Part model, mm, in its own coordinate system. A direction names the side the tool comes from. Coordinates: 2 decimals unless noted, no trailing zeros. Write each loop counter-clockwise with the first axis right and the second up, starting at its lowest first coordinate (ties: lowest second). Pieces come first, ordered by that corner, then holes. Notation, with made-up numbers: (-37.5, -9) -> (8.5, -9) arc R22 cw to (8.5, 12) -> close; hole circle Ø9 at (33, 4). An arc over 180 degrees is marked (long way). One line per question, with ' | ' between items. Start each with the question number.
Item 1: 3-axis set-ups, long thin cutter, end or side, ignore diameter. For faces 1 (the flat face through (77.042, 24.437, 135.393)), 2 (the flat face through (68, 11, 91)): which of +Z, -Z, +X, -X, +Y, -Y reach the whole face in a straight line?
Item 2: Two-plate mould, pull along Y, no slides. Class faces 3 (the cylindrical face through (77.04, 18.35, 147.49)), 4 (the cylindrical face through (77.042, 22.789, 154.427)), 5 (the flat face through (80, 16, 103)): pulls with the +Y half, pulls with the -Y half, needs draft (parallel to the pull), parting line crosses it, or undercut.
Item 3: Saw through at A-A (y = 19.25). List the corners of the cut face in (x, z).
Item 4: Saw through at C-C (y = 25.25). List the corners of the cut face in (x, z), and give its area (3 significant figures).
Item 5: Pin check, flat tips, straight feed: pin 1 (8 mm diameter, centred on x = 63, z = 135.5, fed in from -Y); pin 2 (4 mm diameter, centred on x = 68, z = 115.5, fed in from +Y); pin 3 (12 mm diameter, centred on x = 65, z = 70.5, fed in from -Y); pin 4 (9.5 mm diameter, centred on y = 19.96, z = 144.96, fed in from -X). Stop position of each tip, or through.
Item 6: Probe probe 1 along X at (y, z) = (13, 149); probe 2 along Z at (x, y) = (58.75, 19.75); probe 3 along Y at (x, z) = (64, 130). List the from-to ranges inside material, lowest first. Write a range as [from, to].
Item 7: Saw through at B-B (z = 135.5). List the corners of the cut face in (x, y).
from build123d import *

# Parameters (mm, degrees)
SKETCH014_R      = 3
EXTRUDE013_DEPTH = 6
BOX025_W         = 23
BOX025_H         = 10
BOX025_DEPTH     = 80


with BuildPart() as union_brazo_central:
    # Sketch014 → Extrude013 (new body)
    with BuildSketch(Plane(origin=(0, 0, 0), x_dir=(0, -1, 0), z_dir=(-1, 0, 0))):
        with BuildLine():
            ThreePointArc((-10.900695, 145.407872), (-23.024313, 154.355924), (-27.779278, 140.057671))
            Line((-27.779278, 140.057671), (-20.026942, 129.238365))
            Line((-20.026942, 129.238365), (-11.026942, 129.238365))
            Line((-10.900695, 145.407872), (-11.026942, 129.238365))
        make_face()
        with Locations((-19.957954, 144.958669)):
            Circle(SKETCH014_R, mode=Mode.SUBTRACT)
    extrude(amount=EXTRUDE013_DEPTH)


with BuildPart() as union_brazo_central_1:
    # Extrude013 placement: moved
    add(union_brazo_central.part.moved(Location((63, 0, 0))))


with BuildPart() as main_brazo_central:
    # Box025 → Box025 (new body)
    with BuildSketch(Plane(origin=(57, 11, 52), x_dir=(1, 0, 0), z_dir=(0, 0, 1))):
        with Locations((11.5, 5)):
            Rectangle(BOX025_W, BOX025_H)
    extrude(amount=BOX025_DEPTH)


with BuildPart() as brazo_central:
    # Link017 base: copy of Union brazo central
    add(union_brazo_central_1.part)


with BuildPart() as brazo_central_1:
    # Link017 placement: moved
    add(brazo_central.part.moved(Location((17, 0, 0))))

    # Fusion021: union Union brazo central, main brazo central
    add(union_brazo_central_1.part)
    add(main_brazo_central.part)


solid = brazo_central_1.part
From the geometry:
1) face 1: -Z, +X, -X, +Y | face 2: -Z, +X, -X, -Y
2) face 3: undercut | face 4: parting line crosses it | face 5: needs draft
3) outline: (57, 52) -> (80, 52) -> (80, 142.04) -> (74, 142.04) -> (74, 132) -> (63, 132) -> (63, 142.04) -> (57, 142.04) -> close; (57, 147.87) -> (63, 147.87) -> (63, 154.74) -> (57, 154.74) -> close; (74, 147.87) -> (80, 147.87) -> (80, 154.74) -> (74, 154.74) -> close
4) outline: (57, 136.53) -> (63, 136.53) -> (63, 153.31) -> (57, 153.31) -> close; (74, 136.53) -> (80, 136.53) -> (80, 153.31) -> (74, 153.31) -> close | area: 201 mm2
5) pin 1: y = 10.95 | pin 2: y = 21 | pin 3: y = 11 | pin 4: x = 57
6) probe 1: [57, 63], [74, 80] | probe 2: [52, 141.97], [147.95, 154.78] | probe 3: [11, 21]
7) outline: (57, 10.98) -> (63, 10.98) -> (63, 24.51) -> (57, 24.51) -> close; (74, 10.98) -> (80, 10.98) -> (80, 24.51) -> (74, 24.51) -> close
